```python
from build123d import *

# Parameters (mm, degrees)
SKETCH1_W           = 36
SKETCH1_H           = 28
BOSS_EXTRUDE1_DEPTH = 5
SKETCH2_R           = 1.5
BOSS_EXTRUDE2_DEPTH = 2
SKETCH3_W           = 36
SKETCH3_H           = 28
SKETCH3_R           = 3
CUT_EXTRUDE3_DEPTH  = 2.5


with BuildPart() as part:
    # Sketch1 → Boss-Extrude1 (new body)
    with BuildSketch(Plane(origin=(0, 0, 0), x_dir=(1, 0, 0), z_dir=(0, 1, 0))):
        Rectangle(SKETCH1_W, SKETCH1_H)
    extrude(amount=BOSS_EXTRUDE1_DEPTH)

    # Sketch2 → Boss-Extrude2 (add)
    with BuildSketch(Plane(origin=(0, 5, 0), x_dir=(1, 0, 0), z_dir=(0, 1, 0))):
        with Locations(Location((-14.5, 10, 0), (0, 0, 90))):
            Circle(SKETCH2_R)
        with Locations(Location((-14, -9.993749023, 0), (0, 0, 90))):
            Circle(SKETCH2_R)
        with Locations(Location((12, -10, 0), (0, 0, 90))):
            Circle(SKETCH2_R)
        with Locations(Location((11.499999249, 9.993749004, 0), (0, 0, 90))):
            Circle(SKETCH2_R)
    extrude(amount=BOSS_EXTRUDE2_DEPTH)

    # Sketch3 → Cut-Extrude3 (cut)
    with BuildSketch(Plane(origin=(0, 5, 0), x_dir=(1, 0, 0), z_dir=(0, 1, 0))):
        Rectangle(SKETCH3_W, SKETCH3_H)
        with Locations(Location((11.499999249, 9.993749004, 0), (0, 0, 270))):
            Circle(SKETCH3_R, mode=Mode.SUBTRACT)
        with Locations(Location((12, -10, 0), (0, 0, 270))):
            Circle(SKETCH3_R, mode=Mode.SUBTRACT)
        with Locations(Location((-14, -9.993749023, 0), (0, 0, 270))):
            Circle(SKETCH3_R, mode=Mode.SUBTRACT)
        with Locations(Location((-14.5, 10, 0), (0, 0, 270))):
            Circle(SKETCH3_R, mode=Mode.SUBTRACT)
    extrude(amount=-CUT_EXTRUDE3_DEPTH, mode=Mode.SUBTRACT)


solid = part.part
```
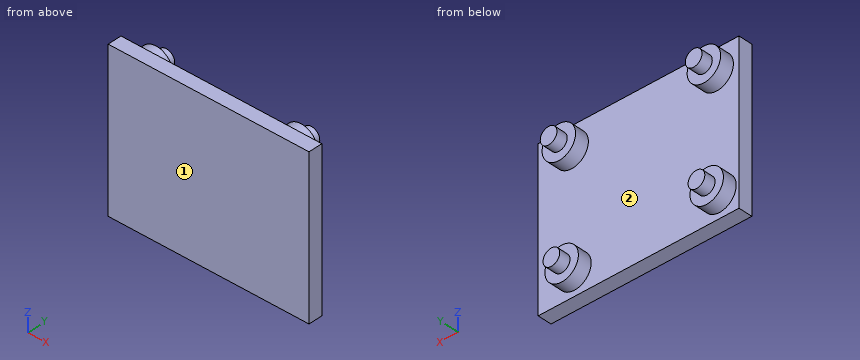
Geometry check sheet. Reference: the model listing, model coordinates, mm. Face numbers are marked on the shaded views. Round coordinates to 2 decimals unless told otherwise and drop trailing zeros. Order: outer loops, then holes, each group sorted by start corner. A loop starts at its lowest first (then second) coordinate and runs counter-clockwise, first axis right, second up. Notation, with made-up numbers: (21.5, 70) - (34.5, 70) arc R24 cw to (34.5, 107) - close; hole circle Ø9 at (38, 13). An arc over 180 degrees is marked (long way). Use a Markdown table: item, result. Add a question column.
1) Section check A-A (y = 6). Record the cut outline in (x, z).
2) Thickness scan on line 1 along X through (y, z) = (5.5, -10); line 2 along Y through (x, z) = (-9.5, 0); line 3 along X through (y, z) = (6, 9.75). Record the ranges inside material, lowest first.
3) Gauge pin test, flat ends, axial feed: P1, Ø6, axis at x = 0.5, z = 2, coming from the -Y side; P2, Ø1, axis at x = -4.5, z = -7, coming from the +Y side; P3, Ø1, axis at x = 10, y = 4, coming from the -Z side. Record the tip position at first contact, or that the pin passes through.
4) Section check C-C (x = -14.5). Record the cut outline in (y, z), then the cut area to 3 significant figures.
5) Mould release check, pull along X, two halves, no side actions. Record for the marked faces 1 and 2: released by +X, released by -X, zero draft, split by the parting line, or undercut.
6) Section check D-D (x = -1). Record the cut outline in (y, z), then the cut area to 3 significant figures.
7) Section check B-B (z = 10). Record the cut outline in (x, y), then the cut area to 3 significant figures.
Established:
| question | item | result |
|---|---|---|
| 1 | outline | circle Ø3 at (-14.5, -10); circle Ø3 at (-14, 9.99); circle Ø3 at (11.5, -9.99); circle Ø3 at (12, 10) |
| 2 | line 1 | -16 to -13, 10 to 13 |
| 2 | line 2 | 0 to 2.5 |
| 2 | line 3 | -15.48 to -12.52, 10.52 to 13.48 |
| 3 | P1 | y = 0 |
| 3 | P2 | y = 2.5 |
| 3 | P3 | z = -12.82 |
| 4 | outline | (0, -14) - (2.5, -14) - (2.5, -13) - (5, -13) - (5, -11.5) - (7, -11.5) - (7, -8.5) - (5, -8.5) - (5, -7) - (2.5, -7) - (2.5, 7.04) - (5, 7.04) - (5, 8.58) - (7, 8.58) - (7, 11.41) - (5, 11.41) - (5, 12.95) - (2.5, 12.95) - (2.5, 14) - (0, 14) - close |
| 4 | area | 111 mm2 |
| 5 | face 1 | zero draft |
| 5 | face 2 | undercut |
| 6 | outline | (0, -14) - (2.5, -14) - (2.5, 14) - (0, 14) - close |
| 6 | area | 70.0 mm2 |
| 7 | outline | (-18, 0) - (18, 0) - (18, 2.5) - (15, 2.5) - (15, 5) - (13.5, 5) - (13.5, 7) - (10.5, 7) - (10.5, 5) - (9, 5) - (9, 2.5) - (-11, 2.5) - (-11, 5) - (-12.5, 5) - (-12.5, 7) - (-15.5, 7) - (-15.5, 5) - (-17, 5) - (-17, 2.5) - (-18, 2.5) - close |
| 7 | area | 132 mm2 |
